For this review, use the dimensioned drawing (mm, ordinates from the lowest corner) and the shaded views. A direction names the side the tool comes from. Coordinates: 2 decimals unless noted, no trailing zeros. Loops run counter-clockwise (first coordinate to the right, second up) from the corner with the lowest first, then second, coordinate; pieces in that order, holes last. Notation, with made-up numbers: (-36.5, -29.75) -> (-28.5, -29.75) arc R29 cw to (-28.5, -3.75) -> close; hole circle Ø4 at (48, -11). An arc over 180 degrees is marked (long way). Use one line per item in the form item = value. Start each with the question number.
1. Wall thickness on line 1 (Y direction, x = 3.5, z = 9.75); line 2 (Y direction, x = 1, z = 11.25) (1 decimal); line 3 (Z direction, x = 5, y = 6.5) (1 decimal): over which ranges is each line inside the solid? List them lowest first. Write a range as from..to.
2. For pin 1 (6 mm diameter, centred on x = 13, z = 12, fed in from -Y); pin 2 (1.5 mm diameter, centred on y = 21.5, z = 6.5, fed in from +X); pin 3 (2 mm diameter, centred on x = 3, y = 17.5, fed in from -Z); pin 4 (6 mm diameter, centred on x = 15.5, y = 17.5, fed in from +Z) (1 decimal), all flat-tipped, find the tip position at first contact; note any pin that passes through.
3. The part is to be moulded in two halves that separate along Y. For the marked faces 1, 2 and 3, say which applies: released by +Y, released by -Y, zero draft, split by the parting line, or undercut.
4. Consider section A-A (y = 2). State the section outline as (x, z) points, then the cut area to 3 significant figures.
5. Machinability: for the marked faces 4 and 5, which of the approach directions +Z, -Z, +X, -X, +Y, -Y give a long, thin tool a straight path to every point of the face, cutting with its end or side? Answer none if there is none.
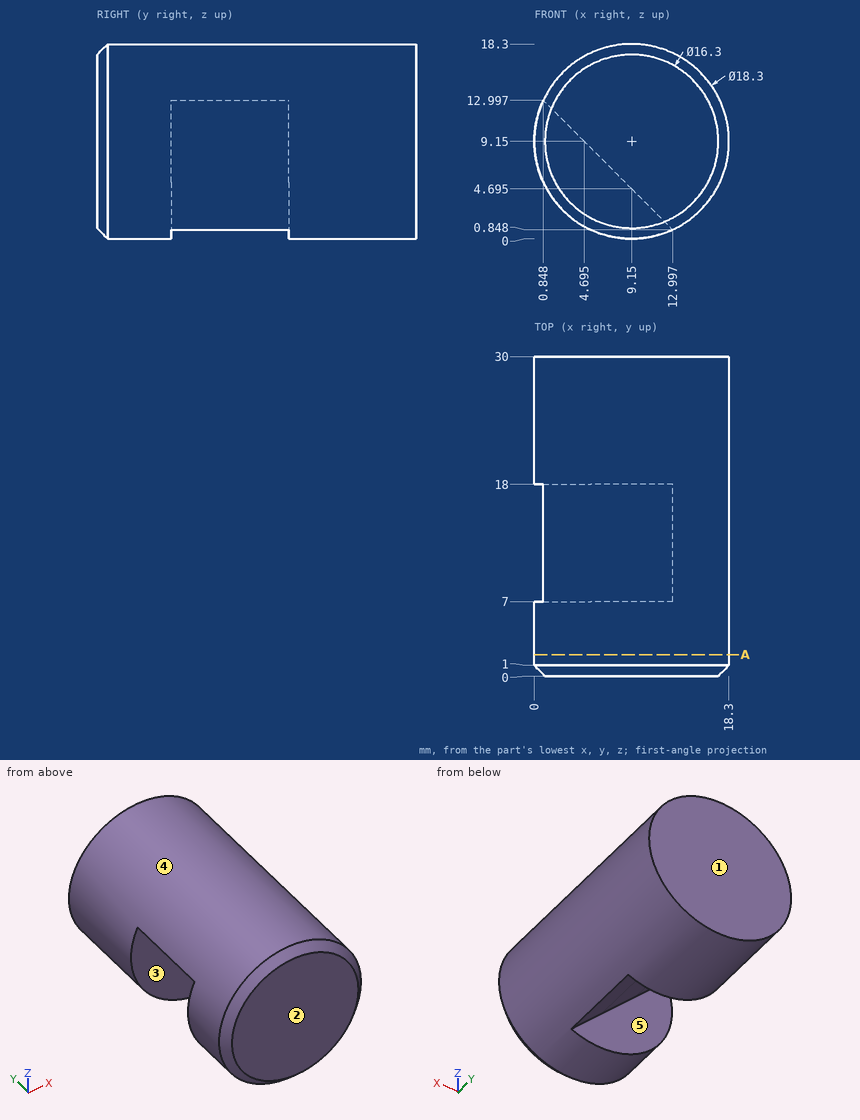
Geometry check:
q1.line_1 = 0..7, 18..30
q1.line_2 = 0.3..7, 18..30
q1.line_3 = 1..17.3
q2.pin_1 = 0
q2.pin_2 = 18.1
q2.pin_3 = 1.68
q2.pin_4 = 17.7
q3.face_1 = released by +Y
q3.face_2 = released by -Y
q3.face_3 = undercut
q4.outline = circle Ø18.3 at (9.15, 9.15)
q4.area = 263 mm²
q5.face_4 = +Y, -Y
q5.face_5 = -Z, -X
